from build123d import *
from OCP.BRepFilletAPI import BRepFilletAPI_MakeChamfer

# Parameters (mm, degrees)
BOSS_EXTRUDE1_DEPTH = 12
SKETCH4_R           = 2.1
CUT_EXTRUDE1_DEPTH  = 27.646669586
CHAMFER1_SIZE       = 2
CHAMFER1_SIZE2      = 1.154700538
FILLET2_R           = 0.75


with BuildPart() as part:
    # Sketch1 → Boss-Extrude1 (new body)
    with BuildSketch(Plane.XY):
        with BuildLine():
            Line((-11.15, 0), (-11.15, -1.5))
            Line((-11.15, -1.5), (-20.15, -1.5))
            Line((-20.15, -1.5), (-20.15, -8.5))
            Line((-20.15, -8.5), (-6.15, -8.5))
            Line((-6.15, -8.5), (-6.15, 0))
            ThreePointArc((-6.15, 0), (0, 6.15), (6.15, 0))
            Line((6.15, 0), (6.15, -8.5))
            Line((6.15, -8.5), (20.15, -8.5))
            Line((20.15, -8.5), (20.15, -1.5))
            Line((20.15, -1.5), (11.15, -1.5))
            Line((11.15, -1.5), (11.15, 0))
            ThreePointArc((11.15, 0), (0, 11.15), (-11.15, 0))
        make_face()
    extrude(amount=BOSS_EXTRUDE1_DEPTH)

    # Sketch4 → Cut-Extrude1 (cut, through all)
    with BuildSketch(Plane(origin=(0, -1.5, 0), x_dir=(1, 0, 0), z_dir=(0, 1, 0))):
        with Locations(Location((-15.65, -6, 0), (0, 0, 180))):
            Circle(SKETCH4_R)
        with Locations(Location((15.65, -6, 0), (0, 0, 180))):
            Circle(SKETCH4_R)
    extrude(amount=-CUT_EXTRUDE1_DEPTH, mode=Mode.SUBTRACT)

    # Chamfer1: one chamfer whose edges measure the first distance from different faces: ONE call of the kernel's chamfer builder (chamfer() names one face for all edges)
    chamfer1_edges_1 = [part.edges().sort_by_distance(p)[0] for p in [
        (-13.55, -1.5, 6),
    ]]
    chamfer1_side_1 = [part.faces().sort_by_distance(p)[0] for p in [
        (-11.3, -1.5, 6),
    ]]
    chamfer1_edges_2 = [part.edges().sort_by_distance(p)[0] for p in [
        (17.75, -1.5, 6),
    ]]
    chamfer1_side_2 = [part.faces().sort_by_distance(p)[0] for p in [
        (20, -1.5, 6),
    ]]
    chamfer1 = BRepFilletAPI_MakeChamfer(part.part.solid().wrapped)
    for e in chamfer1_edges_1:
        chamfer1.Add(CHAMFER1_SIZE, CHAMFER1_SIZE2, e.wrapped, chamfer1_side_1[0].wrapped)  # the first distance lies on this face
    for e in chamfer1_edges_2:
        chamfer1.Add(CHAMFER1_SIZE, CHAMFER1_SIZE2, e.wrapped, chamfer1_side_2[0].wrapped)  # the first distance lies on this face
    add(Compound.cast(chamfer1.Shape()), mode=Mode.REPLACE)

    # Fillet2
    fillet2_edges = [part.edges().sort_by_distance(p)[0] for p in [
        (11.15, -0.75, 0),
        (20.15, -5, 0),
        (-20.15, -5, 0),
        (-11.15, -0.75, 0),
        (0, 11.15, 0),
        (-20.15, -5, 12),
        (20.15, -5, 12),
        (11.15, -0.75, 12),
        (0, 11.15, 12),
        (-11.15, -0.75, 12),
    ]]
    fillet(fillet2_edges, radius=FILLET2_R)


solid = part.part
Part model, mm, in its own coordinate system. A direction names the side the tool comes from. Coordinates: 2 decimals unless noted, no trailing zeros. Order: outer loops, then holes, each group sorted by start corner. A loop starts at its lowest first (then second) coordinate and runs counter-clockwise, first axis right, second up. Notation, with made-up numbers: M 6.5,52.5 L 27.5,52.5 A21 cw 27.5,79.5 Z; hole C 19,9.5 d9. An arc over 180 degrees is marked long. One line per question, with ' | ' between items.
Q1. Drill centre lines: line 1 (Z direction, x = -15.65, y = -7.3); line 2 (Y direction, x = -12, z = 10.75); line 3 (X direction, y = 2.75, z = 2.5). Where is each one in solid material? Low to high.
A:
line 1: z = 0 to 3.9, 8.1 to 12 | line 2: y = -8.5 to -1.5 | line 3: x = -10.81 to -5.5, 5.5 to 10.81
Q2. Slice it at A-A (y = -5.5). Give the cut face in (x, z).
A:
outline: M -20.15,0.75 A0.75 ccw -19.4,0 L -6.15,0 L -6.15,12 L -19.4,12 A0.75 ccw -20.15,11.25 Z; M 6.15,0 L 19.4,0 A0.75 ccw 20.15,0.75 L 20.15,11.25 A0.75 ccw 19.4,12 L 6.15,12 Z; hole C -15.65,6 d4.2; hole C 15.65,6 d4.2
Q3. Slice it at C-C (z = 6). Give the cut face in (x, y).
A:
outline: M -20.15,-8.5 L -17.75,-8.5 L -17.75,-2.65 L -19.75,-1.5 L -20.15,-1.5 Z; M -13.55,-8.5 L -6.15,-8.5 L -6.15,0 A6.15 cw 6.15,0 L 6.15,-8.5 L 13.55,-8.5 L 13.55,-2.65 L 11.55,-1.5 L 11.15,-1.5 L 11.15,0 A11.15 ccw -11.15,0 L -11.15,-1.5 L -11.55,-1.5 L -13.55,-2.65 Z; M 17.75,-8.5 L 20.15,-8.5 L 20.15,-1.5 L 19.75,-1.5 L 17.75,-2.65 Z
Q4. Slice it at B-B (x = -15.65). Give the cut face in (y, z).
A:
outline: M -8.5,0 L -1.5,0 L -1.5,1.9 L -2.65,3.9 L -8.5,3.9 Z; M -8.5,8.1 L -2.65,8.1 L -1.5,10.1 L -1.5,12 L -8.5,12 Z
Q5. 3-axis set-ups, long thin cutter, end or side, ignore diameter. For faces 5 (the face through (6.15, -4, 6)), 6 (the face through (-11.15, -1, 6)), 7 (the face through (11.15, -1, 6)): which of +Z, -Z, +X, -X, +Y, -Y reach the whole face in a straight line?
A:
face 5: +Z, -Z, -Y | face 6: +Z, -Z, -X, +Y | face 7: +Z, -Z, +X, +Y
Q6. Two-plate mould, pull along Z, no slides. Class faces 1 (the face through (17.198, -5.536, 7.419)), 2 (the face through (4, 5, 0)), 3 (the face through (-17.653, -5.536, 6.631)), 4 (the face through (-6.15, -4, 6)): +Z half, -Z half, draft (parallel to the pull), parting line (faces both ways), or undercut.
A:
face 1: undercut | face 2: -Z half | face 3: undercut | face 4: draft
Q7. Pin check, flat tips, straight feed: P1, Ø1, axis at x = 7, y = 3, coming from the -Z side; P2, Ø5, axis at y = 2, z = 5.5, coming from the +X side; P3, Ø8, axis at x = 1, y = 0, coming from the -Z side; P4, Ø3, axis at x = -14, z = 9, coming from the +Y side. Stop position of each tip, or through.
A:
P1: stops at z = 0 | P2: stops at x = 11.15 | P3: passes through | P4: stops at y = -1.5
Q8. Slice it at D-D (z = 1.5). Give the cut face in (x, y), and give its area (3 significant figures).
A:
outline: M -20.15,-8.5 L -6.15,-8.5 L -6.15,0 A6.15 cw 6.15,0 L 6.15,-8.5 L 20.15,-8.5 L 20.15,-1.5 L 11.15,-1.5 L 11.15,0 A11.15 ccw -11.15,0 L -11.15,-1.5 L -20.15,-1.5 Z | area: 347 mm^2
